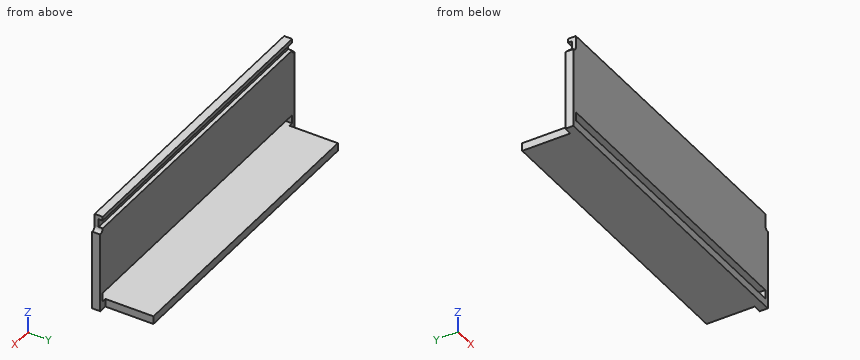
Autodesk Inventor part; units mm, degrees
ref_plane "YZ Plane" through (0, 0, 0) normal (1, 0, 0) x (0, 1, 0)
ref_plane "XZ Plane" through (0, 0, 0) normal (0, 1, 0) x (-1, 0, 0)
ref_plane "XY Plane" through (0, 0, 0) normal (0, 0, 1) x (1, 0, 0)
sketch "Sketch1" plane through (0, 0, 0) normal (0, 1, 0) x (-1, 0, 0)
  line L0 (0, 0) -> (-123.825, 0)
  line L1 (-123.825, 0) -> (-123.825, 38.1)
  line L2 (-123.825, 38.1) -> (0, 38.1)
  line L3 (0, 38.1) -> (0, 0)
  dimension "d0" = 123.825
  dimension "d1" = 38.1
extrude "Extrusion1" add sketch "Sketch1" along normal blind 3.175
sketch "Sketch2" plane through (0, 3.175, 0) normal (0, 1, 0) x (1, 0, 0)
  line L0 (123.825, 0) -> (0, 0)
  line L1 (0, 0) -> (0, -38.1)
  line L2 (0, -38.1) -> (123.825, -38.1)
  line L3 (123.825, -38.1) -> (123.825, 0)
  line L4 (0, -36.5125) -> (123.825, -36.5125)
  line L5 (123.825, -36.5125) -> (123.825, -33.3121)
  line L6 (123.825, -33.3121) -> (0, -33.3121)
  line L7 (0, -33.3121) -> (0, -36.5125)
  line L8 (1.5875, -3.175) -> (87.3125, -3.175)
  line L9 (87.3125, -3.175) -> (87.3125, -6.604)
  line L10 (87.3125, -6.604) -> (1.5875, -6.604)
  line L11 (1.5875, -6.604) -> (1.5875, -3.175)
  dimension "d4" = 3.2004
  dimension "d5" = 1.5875
  dimension "d8" = 85.725
  dimension "d9" = 1.5875
  dimension "d10" = 3.429
  dimension "d11" = 3.175
extrude "Extrusion2" cut sketch "Sketch2" against normal blind 1.5875 contours L3 L4 L1 L6
sketch "Sketch3" plane through (0, 3.175, 0) normal (0, 1, 0) x (1, 0, 0)
  line L0 (123.825, 0) -> (0, 0)
  line L1 (0, 0) -> (0, -33.3121)
  line L2 (1.5875, -3.175) -> (122.2375, -3.175)
  line L3 (122.2375, -3.175) -> (122.2375, -6.604)
  line L4 (122.2375, -6.604) -> (1.5875, -6.604)
  line L5 (1.5875, -6.604) -> (1.5875, -3.175)
  line L6 (123.825, -33.3121) -> (123.825, 0)
  dimension "d15" = 3.429
  dimension "d16" = 3.175
  dimension "d17" = 1.5875
  dimension "d20" = 1.5875
extrude "Extrusion3" cut sketch "Sketch3" against normal blind 12.7
sketch "Sketch4" plane through (0, 3.175, 0) normal (0, 1, 0) x (1, 0, 0)
  line L0 (0, -38.1) -> (1.5875, -38.1)
  line L1 (1.5875, -38.1) -> (1.5875, -31.75)
  line L2 (1.5875, -31.75) -> (0, -31.75)
  line L3 (0, -31.75) -> (0, -38.1)
  line L4 (123.825, -38.1) -> (122.2375, -38.1)
  line L5 (122.2375, -38.1) -> (122.2375, -31.75)
  line L6 (122.2375, -31.75) -> (123.825, -31.75)
  line L7 (123.825, -31.75) -> (123.825, -38.1)
  point P0 (0, 0)
  dimension "d21" = 1.5875
  dimension "d22" = 6.35
  dimension "d23" = 6.35
  dimension "d24" = 1.5875
extrude "Extrusion4" cut sketch "Sketch4" against normal blind 12.7
fillet "Fillet1" radius 1.5875 2 edges at (122.2375, 1.5875, 31.75) (1.5875, 1.5875, 31.75)
sketch "Sketch5" plane through (0, 3.175, 0) normal (0, 1, 0) x (1, 0, 0)
  line L0 (123.825, -31.75) -> (123.825, 0)
  line L1 (3.2004, 0) -> (120.6246, 0)
  line L2 (120.6246, 0) -> (120.6246, -3.175)
  line L3 (120.6246, -3.175) -> (3.2004, -3.175)
  line L4 (3.2004, -3.175) -> (3.2004, 0)
  line L5 (0, 0) -> (0, -31.75)
  dimension "d31" = 3.175
  dimension "d32" = 3.2004
  dimension "d33" = 3.2004
extrude "Extrusion5" add sketch "Sketch5" along normal blind 19.05
properties part number "Electronics Container Part 5"
Read the model definition and answer for the solid it produces. Units are mm, in the model's axes. Give positions to 0.01 mm unless a question says otherwise; leave off trailing zeros. Write each loop counter-clockwise with the first axis right and the second up, starting at its lowest first coordinate (ties: lowest second). Pieces come first, ordered by that corner, then holes. Notation, with made-up numbers: (-7, 17.5) - (-1, 17.5) arc R33 ccw to (-1, 55.5) - close; hole circle Ø9 at (-19.5, 1). An arc over 180 degrees is marked (long way). Answer in a Markdown table with one row per item. Add a question column.
Item 1: Section A-A, the plane x = 12.5 is taken. Write down the section's boundary in (y, z) (1 decimal), and give its area (3 significant figures).
Item 2: Flat-ended cylindrical pins translate along their axes: P1, Ø1.5, axis at x = 91, y = 13, coming from the +Z side (3 decimals); P2, Ø1.3, axis at x = 42.5, z = 37, coming from the +Y side (3 decimals); P3, Ø1.6, axis at y = 1, z = 35.5, coming from the -X side. Find the tip coordinate at first contact, or state that the pin passes through.
Item 3: Section C-C, the plane y = 11.25 is taken. Write down the section's boundary in (x, z) (3 decimals), and give its area (3 significant figures).
Item 4: Section B-B, the plane z = 12 is taken. Write down the section's boundary in (x, y) (3 decimals), and give its area (3 significant figures).
Item 5: Find the intervals of material crossed by L1, parallel to Z at x = 84, y = 3 (1 decimal); L2, parallel to Y at x = 68, z = 14 (3 decimals), in increasing order.
Recorded:
| question | item | result |
|---|---|---|
| 1 | outline | (0, 0) - (22.2, 0) - (22.2, 3.2) - (0, 3.2) - close; (0, 6.6) - (3.2, 6.6) - (3.2, 33.3) - (1.6, 33.3) - (1.6, 36.5) - (3.2, 36.5) - (3.2, 38.1) - (0, 38.1) - close |
| 1 | area | 165 mm2 |
| 2 | P1 | stops at z = 3.175 |
| 2 | P2 | stops at y = 3.175 |
| 2 | P3 | stops at x = 1.59 |
| 3 | outline | (3.2, 0) - (120.625, 0) - (120.625, 3.175) - (3.2, 3.175) - close |
| 3 | area | 373 mm2 |
| 4 | outline | (0, 0) - (123.825, 0) - (123.825, 3.175) - (0, 3.175) - close |
| 4 | area | 393 mm2 |
| 5 | L1 | z = 0 to 3.2, 6.6 to 33.3, 36.5 to 38.1 |
| 5 | L2 | y = 0 to 3.175 |
